from build123d import *

# Parameters (mm, degrees)
SKETCH_5_W          = 70
SKETCH_5_H          = 70
EXTRUDE_2_DEPTH     = 130
SKETCH_11_R         = 27.5
EXTRUDE_4_DEPTH     = 1525
SKETCH_12_W         = 103.923048454
SKETCH_12_H         = 8.094806624
SKETCH_12_H_2       = 10.367731853
CUT_EXTRUDE_1_DEPTH = 75
CUT_EXTRUDE_START   = -75
SKETCH_13_R         = 30
CUT_EXTRUDE_2_DEPTH = 75
FILLET_3_R          = 5
FILLET_2_R          = 1
CHAMFER_2_SIZE      = 1


with BuildPart() as part:
    # 草图3 → 旋转1 (revolve)
    with BuildSketch(Plane.XY):
        with BuildLine():
            Line((-30, -30), (-30, 30))
            Line((-30, 30), (-51.961524227, 30))
            ThreePointArc((-51.961524227, 30), (-60, 0), (-51.961524227, -30))
            Line((-51.961524227, -30), (-30, -30))
        make_face()
    revolve(axis=Axis((0, 0, 0), (0, 1, 0)))

    # 草图5 → 凸台-拉伸2 (add)
    with BuildSketch(Plane.XY.offset(-130)):
        Rectangle(SKETCH_5_W, SKETCH_5_H)
    extrude(amount=EXTRUDE_2_DEPTH)

    # 草图11 → 凸台-拉伸4 (add)
    with BuildSketch(Plane(origin=(0, 0, -130), x_dir=(-1, 0, 0), z_dir=(0, 0, -1))):
        Circle(SKETCH_11_R)
    extrude(amount=EXTRUDE_4_DEPTH)

    # 草图12 → 切除-拉伸1 (cut)
    with BuildSketch(Plane.XY):
        with Locations((0, 34.047403312)):
            Rectangle(SKETCH_12_W, SKETCH_12_H)
        with Locations((0, -35.183865927)):
            Rectangle(SKETCH_12_W, SKETCH_12_H_2)
    extrude(amount=-CUT_EXTRUDE_1_DEPTH, mode=Mode.SUBTRACT)

    # 草图13 → 切除-拉伸2 (cut)
    with BuildSketch(Plane.XZ.offset(30).offset(CUT_EXTRUDE_START)):
        with Locations(Location((0, 0, 0), (0, 0, 270))):
            Circle(SKETCH_13_R)
    extrude(amount=CUT_EXTRUDE_2_DEPTH, mode=Mode.SUBTRACT)

    # 圆角3
    fillet_3_edges = [part.edges().sort_by_distance(p)[0] for p in [
        (0, -30, -75),
        (0, 30, -75),
    ]]
    fillet(fillet_3_edges, radius=FILLET_3_R - 0.0001)  # a hair under: the kernel refuses the full size

    # 圆角2
    fillet_2_edges = [part.edges().sort_by_distance(p)[0] for p in [
        (27.5, 0, -130),
    ]]
    fillet(fillet_2_edges, radius=FILLET_2_R)

    # 倒角2
    chamfer_2_edges = [part.edges().sort_by_distance(p)[0] for p in [
        (35, 0, -130),
        (-35, 0, -130),
        (0, 35, -130),
        (0, -35, -130),
    ]]
    chamfer(chamfer_2_edges, length=CHAMFER_2_SIZE)


solid = part.part
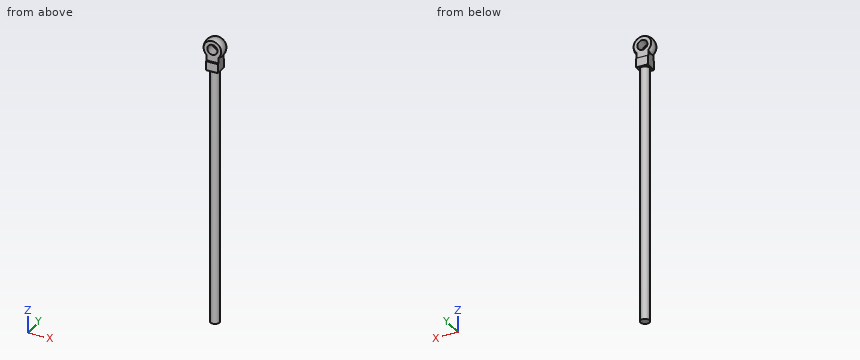
The listing builds one solid part. Answer for the finished solid, in the listing's coordinates (mm). Round coordinates to 2 decimals unless told otherwise and drop trailing zeros. Write each loop counter-clockwise with the first axis right and the second up, starting at its lowest first coordinate (ties: lowest second). Pieces come first, ordered by that corner, then holes. Notation, with made-up numbers: M 56.5,29.5 L 76.5,29.5 A13 ccw 76.5,53.5 Z; hole C 20.25,64.5 d8. An arc over 180 degrees is marked long. Write each question's results on one line, items separated by ' | '. Start each with the question number.
Item 1: Given pin 1 Ø1.5 at (x, z) = (5, -913) entering from -Y; pin 2 Ø1 at (x, y) = (-29.5, 10) entering from +Z; pin 3 Ø12 at (x, y) = (12.5, 6) entering from +Z, each flat-ended and moving along its own axis, determine where each tip first touches the part or whether it passes through.
Item 2: Straight lines are drawn through the part: probe 1 along X at (y, z) = (-5, 0); probe 2 along Z at (x, y) = (0, 0); probe 3 along X at (y, z) = (1, 0). For each, find the intervals that lie inside material, in ascending order.
Item 3: Find section A-A on z = 0. Write down the section's boundary in (x, y).
Item 4: Find section C-C on y = 0. Write down the section's boundary in (x, z), and give its area (3 significant figures).
Item 5: Find section D-D on z = -1244.5. Write down the section's boundary in (x, y), and give its area (3 significant figures).
Answer block:
1) pin 1: stops at y = -27.17 | pin 2: stops at z = 51.58 | pin 3: stops at z = 59.48
2) probe 1: x = -59.79 to -30, 30 to 59.79 | probe 2: z = -1655 to -30, 30 to 60 | probe 3: x = -59.99 to -30, 30 to 59.99
3) outline: M -51.96,-30 L -30,-30 L -30,30 L -51.96,30 A60 ccw Z; M 30,-30 L 51.96,-30 A60 ccw 51.96,30 L 30,30 Z
4) outline: M -35,-129 L -34,-130 L -28.5,-130 A1 cw -27.5,-131 L -27.5,-1655 L 27.5,-1655 L 27.5,-131 A1 cw 28.5,-130 L 34,-130 L 35,-129 L 35,-48.73 A60 ccw long -35,-48.73 Z; hole C 0,0 d60 | area: 97,500 mm²
5) outline: C 0,0 d55 | area: 2,380 mm²
